Geometry check sheet. Reference: drawing and pictorial views, mm from the part's lowest x, y, z. Give positions to 0.01 mm unless a question says otherwise; leave off trailing zeros. Loops run counter-clockwise (first coordinate to the right, second up) from the corner with the lowest first, then second, coordinate; pieces in that order, holes last. Notation, with made-up numbers: (-23, 39) - (16, 39) arc R13 ccw to (16, 62) - close; hole circle Ø2 at (30, -9.5). An arc over 180 degrees is marked (long way). Answer in a Markdown table with one row per item. Add a question column.
(1) Sectioned sample at A-A on x = 11.5. Enter the section's corners in (y, z) (1 decimal), then the cut area to 3 significant figures.
(2) Sectioned sample at C-C on y = 39.5. Enter the section's corners in (x, z) (1 decimal).
(3) Sectioned sample at B-B on z = 0.55. Enter the section's corners in (x, y) (1 decimal), then the cut area to 3 significant figures.
(4) Sectioned sample at D-D on x = 42.5. Enter the section's corners in (y, z) (1 decimal).
(5) Thickness scan on L1, parallel to X at y = 39, z = 0.7 (1 decimal); L2, parallel to X at y = 89, z = 0.25 (1 decimal); L3, parallel to Y at x = 48, z = 0.4. Record the ranges inside material, lowest first.
(6) Go/stop test with flat-tipped pins: P1, Ø0.5, axis at y = 31.5, z = 1, coming from the +X side; P2, Ø0.5, axis at x = 4, z = 0.5, coming from the +Y side; P3, Ø0.8, axis at x = 1, z = 1, coming from the -Y side. Record where each tip stops, or that it passes through.
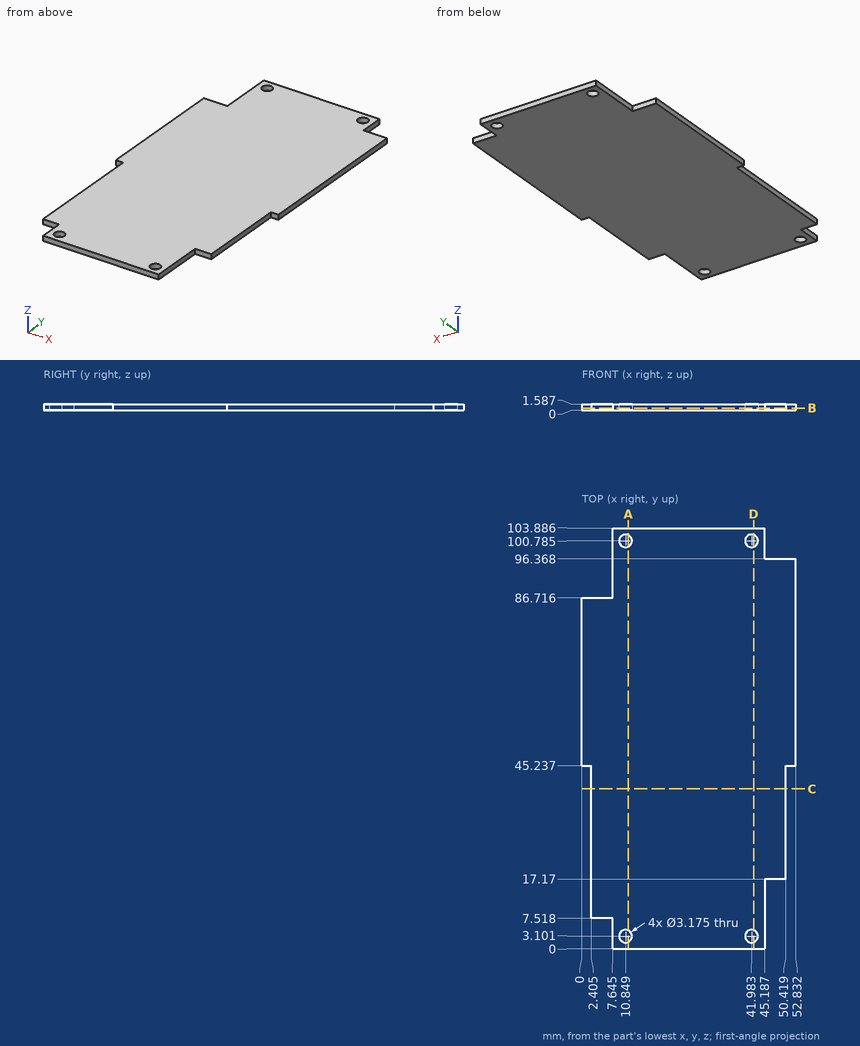
Reply:
| question | item | result |
|---|---|---|
| 1 | outline | (0, 0) - (1.7, 0) - (1.7, 1.6) - (0, 1.6) - close; (4.5, 0) - (99.3, 0) - (99.3, 1.6) - (4.5, 1.6) - close; (102.2, 0) - (103.9, 0) - (103.9, 1.6) - (102.2, 1.6) - close |
| 1 | area | 156 mm^2 |
| 2 | outline | (2.4, 0) - (50.4, 0) - (50.4, 1.6) - (2.4, 1.6) - close |
| 3 | outline | (0, 45.2) - (2.4, 45.2) - (2.4, 7.5) - (7.6, 7.5) - (7.6, 0) - (45.2, 0) - (45.2, 17.2) - (50.4, 17.2) - (50.4, 45.2) - (52.8, 45.2) - (52.8, 96.4) - (45.2, 96.4) - (45.2, 103.9) - (7.6, 103.9) - (7.6, 86.7) - (0, 86.7) - close; hole circle Ø3.2 at (10.8, 3.1); hole circle Ø3.2 at (10.8, 100.8); hole circle Ø3.2 at (42, 3.1); hole circle Ø3.2 at (42, 100.8) |
| 3 | area | 4,920 mm^2 |
| 4 | outline | (0, 0) - (1.6, 0) - (1.6, 1.6) - (0, 1.6) - close; (4.6, 0) - (99.3, 0) - (99.3, 1.6) - (4.6, 1.6) - close; (102.3, 0) - (103.9, 0) - (103.9, 1.6) - (102.3, 1.6) - close |
| 5 | L1 | 2.4 to 50.4 |
| 5 | L2 | 7.6 to 52.8 |
| 5 | L3 | 17.17 to 96.37 |
| 6 | P1 | x = 50.42 |
| 6 | P2 | y = 86.72 |
| 6 | P3 | y = 45.24 |
